The listing builds one solid part. Answer for the finished solid, in the listing's coordinates (mm). Face numbers are marked on the shaded views. A direction names the side the tool comes from. Round coordinates to 2 decimals unless told otherwise and drop trailing zeros. Order: outer loops, then holes, each group sorted by start corner. A loop starts at its lowest first (then second) coordinate and runs counter-clockwise, first axis right, second up. Notation, with made-up numbers: (61.5, 60) - (104.5, 60) arc R19 ccw to (104.5, 75) - close; hole circle Ø1 at (84, -38.5). An arc over 180 degrees is marked (long way). Use CSV: the item, a comma, the result in double quotes. Start each with the question number.
Item 1: For the marked faces 4 and 5, determine the directions among +Z, -Z, +X, -X, +Y, -Y from which every point of the face is accessible in a straight line to the end or side of a thin tool.
Item 2: Flat-ended cylindrical pins translate along their axes: P1, Ø4.5, axis at x = 1, z = 4, coming from the -Y side; P2, Ø1.1, axis at y = -267, z = -12.5, coming from the +X side; P3, Ø3, axis at x = 0, z = -11.5, coming from the -Y side. Find the tip coordinate at first contact, or state that the pin passes through.
Item 3: Find section C-C, the plane y = -64.5. Give the vertices of the cut face in (x, z), plus the area to 3 significant figures.
Item 4: Determine the mould class of the marked faces 1, 2 and 3 for opening direction Z: +Z half, -Z half, draft (parallel to the pull), parting line (faces both ways), or undercut.
Item 5: Find section A-A, the plane x = 0. Give the vertices of the cut face in (y, z), plus the area to 3 significant figures.
Item 6: Find section B-B, the plane y = -242.5. Give the vertices of the cut face in (x, z), plus the area to 3 significant figures.
Item 7: Straight lines are drawn through the part: line 1 along Z through (x, y) = (-1, -238); line 2 along Y through (x, z) = (22, 2.5); line 3 along Z through (x, y) = (1, -113.5). For each, find the intervals that lie inside material, in ascending order. Write a range as [from, to].
```python
from build123d import *

# Parameters (mm, degrees)
F0_R      = 24.0021072249
F1_DEPTH  = 177.8
F2_R      = 5.2565656239
F2_R_2    = 5.5580260463
F3_DEPTH  = 76.2
F4_R      = 2.5394375709
F4_R_2    = 3.0260152953
F5_DEPTH  = 25.4
F6_R      = 1.4824915772
F6_R_2    = 1.4854629447
F7_DEPTH  = 12.7
F8_W      = 9.9838948809
F8_H      = 8.7704055477
F9_DEPTH  = 10.16
F10_R     = 2.6763905771
F11_DEPTH = 63.5
F12_R     = 6.2569040354
F13_DEPTH = 76.2
F14_W     = 6.9022711832
F14_H     = 3.66242975
F15_DEPTH = 25.4
F16_R     = 6.2007059651
F17_DEPTH = 76.2


# Not quite as in the source:
# - a length typed as a fraction of an inch, garbled in the dataset ("3 / 203.2 mm" for 3/8 in), is restored


with BuildPart() as f1:
    # F0 (on Front) → F1 (new body)
    with BuildSketch(Plane.XZ):
        Circle(F0_R)
    extrude(amount=F1_DEPTH)

    # F2 (on face) → F3 (join)
    with BuildSketch(Plane.XZ.offset(177.8)):
        with Locations((-14.8806795478, 0)):
            Circle(F2_R)
        with Locations((14.4999595359, 0)):
            Circle(F2_R_2)
    extrude(amount=F3_DEPTH)

    # F4 (on face) → F5 (join)
    with BuildSketch(Plane.XZ.offset(254)):
        with Locations((-15.0723066181, 0)):
            Circle(F4_R)
        with Locations((14.4999595359, 0)):
            Circle(F4_R_2)
    extrude(amount=F5_DEPTH)

    # F6 (on face) → F7 (join)
    with BuildSketch(Plane.XZ.offset(279.4)):
        with Locations((-15.0723066181, 0)):
            Circle(F6_R)
        with Locations((14.5250931382, 0)):
            Circle(F6_R_2)
    extrude(amount=F7_DEPTH)

    # F8 (on face) → F9 (join)
    with BuildSketch(Plane.XZ.offset(177.8)):
        with Locations((0.2944918815, 2.0464671543)):
            Rectangle(F8_W, F8_H)
    extrude(amount=F9_DEPTH)

    # F10 (on face) → F11 (join)
    with BuildSketch(Plane.XZ.offset(187.96)):
        with Locations((0, 2.6763908099)):
            Circle(F10_R)
    extrude(amount=F11_DEPTH)

    # F12 (on face) → F13 (join)
    with BuildSketch(Plane.XZ.offset(177.8)):
        with Locations((0, -12.9593666643)):
            Circle(F12_R)
    extrude(amount=F13_DEPTH)

    # F14 (on face) → F15 (join)
    with BuildSketch(Plane.XZ.offset(254)):
        with Locations((-0.0704309205, -11.6916019469)):
            Rectangle(F14_W, F14_H)
    extrude(amount=F15_DEPTH)

    # F16 (on face) → F17 (join)
    with BuildSketch(Plane.XZ.offset(177.8)):
        with Locations((0, 15.626385808)):
            Circle(F16_R)
    extrude(amount=F17_DEPTH)


solid = f1.part
```
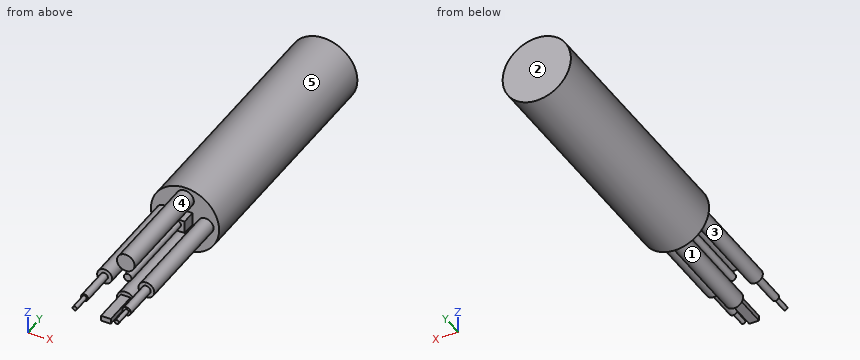
Worked out:
1,face 4,"-Y"
1,face 5,"+Y, -Y"
2,P1,"stops at y = -251.46"
2,P2,"stops at x = 3.38"
2,P3,"stops at y = -279.4"
3,outline,"circle Ø48 at (0, 0)"
3,area,"1,810 mm²"
4,face 1,"undercut"
4,face 2,"draft"
4,face 3,"parting line"
5,outline,"(-279.4, -13.52) - (-254, -13.52) - (-254, -19.22) - (-177.8, -19.22) - (-177.8, -24) - (0, -24) - (0, 24) - (-177.8, 24) - (-177.8, 21.83) - (-254, 21.83) - (-254, 9.43) - (-177.8, 9.43) - (-177.8, 6.43) - (-187.96, 6.43) - (-187.96, 5.35) - (-251.46, 5.35) - (-251.46, 0) - (-187.96, 0) - (-187.96, -2.34) - (-177.8, -2.34) - (-177.8, -6.7) - (-254, -6.7) - (-254, -9.86) - (-279.4, -9.86) - close"
5,area,"11,000 mm²"
6,outline,"circle Ø10.51 at (-14.88, 0); circle Ø12.51 at (0, -12.96); circle Ø12.4 at (0, 15.63); circle Ø5.35 at (0, 2.68); circle Ø11.12 at (14.5, 0)"
6,area,"450 mm²"
7,line 1,"z = [-19.14, -6.78], [0.19, 5.16], [9.51, 21.75]"
7,line 2,"y = [-177.8, 0]"
7,line 3,"z = [-23.98, 23.98]"
